Can you work these out from the model? Positions are in its coordinate system, mm. A direction names the side the tool comes from. Coordinates: 2 decimals unless noted, no trailing zeros. Loops run counter-clockwise (first coordinate to the right, second up) from the corner with the lowest first, then second, coordinate; pieces in that order, holes last. Notation, with made-up numbers: (5.5, -24) -> (47.5, -24) arc R14 ccw to (47.5, -1) -> close; hole circle Ø9 at (65.25, -35). An arc over 180 degrees is marked (long way). Use one line per item in the form item = value. Start each with the question number.
(1) Imagine slicing it at D-D (z = 2.25). List the corners of the cut face in (x, y) for me, plus the area to 3 significant figures.
(2) I'm going to push flat-ended pins straight in: pin 1 (1 mm diameter, centred on y = 5, z = 9, fed in from -X); pin 2 (11 mm diameter, centred on x = 1.5, y = 4.5, fed in from -Z); pin 3 (2 mm diameter, centred on y = 0.5, z = 8.5, fed in from -X); pin 4 (14.5 mm diameter, centred on x = 0, y = 0, fed in from -Z). Where does each tip first touch, or does it pass through?
(3) On a 3-axis mill with a long thin cutter (end or side, diameter ignored), from which of +Z, -Z, +X, -X, +Y, -Y can I reach the whole of each face in a straight line? I mean faces 4 (the flat face through (25, -19, 5)), 5 (the flat face through (-2, -9, 6)), 6 (the flat face through (-20, -15, 5)). Say none if no direction works.
(4) Imagine slicing it at C-C (x = -4.5). List the corners of the cut face in (y, z) for me.
(5) Imagine slicing it at B-B (y = 0). List the corners of the cut face in (x, z) for me, plus the area to 3 significant figures.
(6) Thinking about a two-plate mould opening in Y: for faces 1 (the cylindrical face through (2.38, -10.74, 2.96)), 2 (the flat face through (20, -15, 5)), 3 (the cylindrical face through (-21.31, -20.07, 4)), which applies, released by +Y, released by -Y, zero draft, split by the parting line, or undercut?
(7) I need wall thicknesses on line 1 (Z direction, x = -20, y = -20.5); line 2 (Y direction, x = 0, z = 2.65); line 3 (Y direction, x = 0, z = 8.6). Which ranges of each line are inside material? Lowest first, please. Write a range as [from, to].
(8) Imagine slicing it at A-A (z = 9.25). List the corners of the cut face in (x, y) for me.
```python
from build123d import *

# Parameters (mm, degrees)
EXTRUDE_1_DEPTH     = 10
SKETCH_2_R          = 11
CUT_EXTRUDE_1_DEPTH = 6
SKETCH_3_R          = 1.65
CUT_EXTRUDE_2_DEPTH = 10
SKETCH_4_R          = 9
CUT_EXTRUDE_3_DEPTH = 36.860842154
FILLET_1_R          = 2


with BuildPart() as part:
    # ｽｹｯﾁ1 → ﾎﾞｽ - 押し出し1 (new body)
    with BuildSketch(Plane.XY):
        with BuildLine():
            Line((-25, -15), (-16.20863824, 6.597730399))
            ThreePointArc((-16.20863824, 6.597730399), (-14.32427611, 10.053114638), (-11.715374514, 13))
            Line((-11.715374514, 13), (11.715374514, 13))
            ThreePointArc((11.715374514, 13), (14.32427611, 10.053114638), (16.20863824, 6.597730399))
            Line((16.20863824, 6.597730399), (25, -15))
            Line((25, -15), (25, -25))
            Line((25, -25), (-25, -25))
            Line((-25, -25), (-25, -15))
        make_face()
    extrude(amount=EXTRUDE_1_DEPTH)

    # ｽｹｯﾁ2 → ｶｯﾄ - 押し出し1 (cut)
    with BuildSketch(Plane(origin=(0, 0, 0), x_dir=(-1, 0, 0), z_dir=(0, 0, -1))):
        Circle(SKETCH_2_R)
    extrude(amount=-CUT_EXTRUDE_1_DEPTH, mode=Mode.SUBTRACT)

    # ｽｹｯﾁ3 → ｶｯﾄ - 押し出し2 (cut)
    with BuildSketch(Plane.XZ.offset(25)):
        with Locations((-20, 5)):
            Circle(SKETCH_3_R)
        with Locations(Location((20, 5, 0), (0, 0, 180))):
            Circle(SKETCH_3_R)
    extrude(amount=-CUT_EXTRUDE_2_DEPTH, mode=Mode.SUBTRACT)

    # ｽｹｯﾁ4 → ｶｯﾄ - 押し出し3 (cut, through all)
    with BuildSketch(Plane(origin=(0, 0, 6), x_dir=(-1, 0, 0), z_dir=(0, 0, -1))):
        Circle(SKETCH_4_R)
    extrude(amount=-CUT_EXTRUDE_3_DEPTH, mode=Mode.SUBTRACT)

    # ﾌｨﾚｯﾄ1
    fillet_1_edges = [part.edges().sort_by_distance(p)[0] for p in [
        (25, -25, 5),
        (-25, -25, 5),
        (-25, -15, 5),
        (-11.715374514, 13, 5),
        (11.715374514, 13, 5),
        (25, -15, 5),
    ]]
    fillet(fillet_1_edges, radius=FILLET_1_R)


solid = part.part
```
Worked out:
q1.outline = (-25, -23) arc R2 ccw to (-23, -25) -> (23, -25) arc R2 ccw to (25, -23) -> (25, -15.39) arc R2 ccw to (24.85, -14.64) -> (16.21, 6.6) arc R17.5 ccw to (12.33, 12.42) arc R2 ccw to (10.92, 13) -> (-10.92, 13) arc R2 ccw to (-12.33, 12.42) arc R17.5 ccw to (-16.21, 6.6) -> (-24.85, -14.64) arc R2 ccw to (-25, -15.39) -> close; hole circle Ø22 at (0, 0)
q1.area = 1,190 mm2
q2.pin_1 = -17.06
q2.pin_2 = 6
q2.pin_3 = -19.1
q2.pin_4 = through
q3.face_4 = +Z, -Z, +X, +Y, -Y
q3.face_5 = -Z
q3.face_6 = -Y
q4.outline = (-25, 0) -> (-10.04, 0) -> (-10.04, 6) -> (-7.79, 6) -> (-7.79, 10) -> (-25, 10) -> close; (7.79, 6) -> (10.04, 6) -> (10.04, 0) -> (13, 0) -> (13, 10) -> (7.79, 10) -> close
q5.outline = (-18.89, 0) -> (-11, 0) -> (-11, 6) -> (-9, 6) -> (-9, 10) -> (-18.89, 10) -> close; (9, 6) -> (11, 6) -> (11, 0) -> (18.89, 0) -> (18.89, 10) -> (9, 10) -> close
q5.area = 174 mm2
q6.face_1 = undercut
q6.face_2 = released by -Y
q6.face_3 = zero draft
q7.line_1 = [0, 3.35], [6.65, 10]
q7.line_2 = [-25, -11], [11, 13]
q7.line_3 = [-25, -9], [9, 13]
q8.outline = (-25, -23) arc R2 ccw to (-23, -25) -> (23, -25) arc R2 ccw to (25, -23) -> (25, -15.39) arc R2 ccw to (24.85, -14.64) -> (16.21, 6.6) arc R17.5 ccw to (12.33, 12.42) arc R2 ccw to (10.92, 13) -> (-10.92, 13) arc R2 ccw to (-12.33, 12.42) arc R17.5 ccw to (-16.21, 6.6) -> (-24.85, -14.64) arc R2 ccw to (-25, -15.39) -> close; hole circle Ø18 at (0, 0)
